Input: part model. Units: mm. Frame: model coordinates. Coordinates: 2 decimals unless noted, no trailing zeros. Write each loop counter-clockwise with the first axis right and the second up, starting at its lowest first coordinate (ties: lowest second). Pieces come first, ordered by that corner, then holes. Notation, with made-up numbers: (-3, 36) - (32, 36) arc R29 ccw to (32, 69) - close; hole circle Ø11 at (-16.5, 42.25). An arc over 180 degrees is marked (long way). Use CSV: the item, a comma, the result in double quotes.
```python
from build123d import *

# Parameters (mm, degrees)
SKETCH1_W           = 37.3
SKETCH1_H           = 400
BOSS_EXTRUDE1_DEPTH = 6.35
SKETCH10_W          = 6.35
SKETCH10_H          = 10
BOSS_EXTRUDE3_DEPTH = 6.35
SKETCH11_W          = 6.35
SKETCH11_H          = 10
BOSS_EXTRUDE4_DEPTH = 6.35
LPATTERN5_COUNT     = 20
LPATTERN5_PITCH     = 20
SKETCH12_W          = 10
SKETCH12_H          = 6.35
BOSS_EXTRUDE5_DEPTH = 6.35


with BuildPart() as part:
    # Sketch1 → Boss-Extrude1 (new body)
    with BuildSketch(Plane.XY):
        Rectangle(SKETCH1_W, SKETCH1_H)
    extrude(amount=BOSS_EXTRUDE1_DEPTH)

    # Sketch10 → Boss-Extrude3 (add)
    with BuildSketch(Plane.XY):
        with Locations((-21.825, -195)):
            Rectangle(SKETCH10_W, SKETCH10_H)
    boss_extrude3 = extrude(amount=BOSS_EXTRUDE3_DEPTH)

    # Sketch11 → Boss-Extrude4 (add)
    with BuildSketch(Plane.XY):
        with Locations((21.825, -185)):
            Rectangle(SKETCH11_W, SKETCH11_H)
    boss_extrude4 = extrude(amount=BOSS_EXTRUDE4_DEPTH)

    # LPattern5: Boss-Extrude3, Boss-Extrude4 ×20
    with Locations(*[(0, i * LPATTERN5_PITCH, 0) for i in range(1, LPATTERN5_COUNT)]):
        add(boss_extrude3)
        add(boss_extrude4)

    # Sketch12 → Boss-Extrude5 (add)
    with BuildSketch(Plane.XY):
        with Locations((0, 203.175)):
            Rectangle(SKETCH12_W, SKETCH12_H)
    boss_extrude5 = extrude(amount=BOSS_EXTRUDE5_DEPTH)

    # Mirror1: Boss-Extrude5 across plane
    add(boss_extrude5.mirror(Plane.ZX))


solid = part.part
```
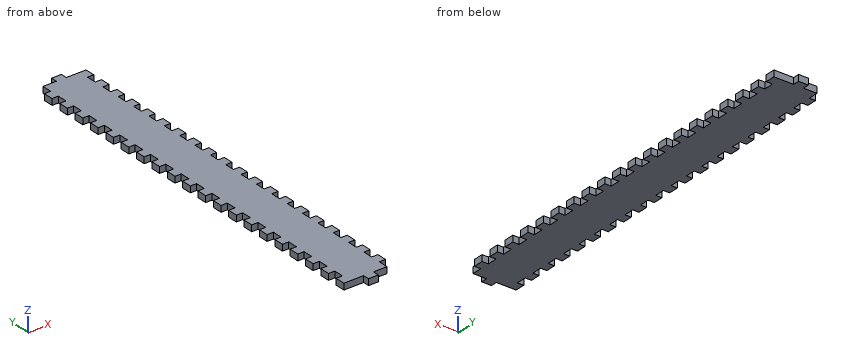
(1) Cut plane A-A on y = -146. Return loops of the section in (x, z).
Check values:
outline,"(-18.65, 0) - (25, 0) - (25, 6.35) - (-18.65, 6.35) - close"
(2) Pin query (flat end, axial travel): pin 1 Ø2 at (x, z) = (-20, 1) entering from +Y; pin 2 Ø1.9 at (x, z) = (21.5, 4.5) entering from -Y; pin 3 Ø3 at (x, z) = (-21, 3) entering from -Y. Return the tip coordinate at first contact, or that it passes through.
Check values:
pin 1,"y = 190"
pin 2,"y = -190"
pin 3,"y = -200"
(3) Cut plane B-B on x = 11.5. Return loops of the section in (y, z), and give its area (3 significant figures).
Check values:
outline,"(-200, 0) - (200, 0) - (200, 6.35) - (-200, 6.35) - close"
area,"2,540 mm^2"
(4) Ray query, probe 1 along Y at (x, z) = (17.5, 4); probe 2 along X at (y, z) = (18, 5.5); probe 3 along X at (y, z) = (-76, 1.5). Return the intervals inside material, ascending. Write a range as from..to.
Check values:
probe 1,"-200..200"
probe 2,"-18.65..25"
probe 3,"-25..18.65"
